```python
from build123d import *

# Parameters (mm, degrees)
BOSS_EXTRUDE1_DEPTH      = 65.5
CUT_EXTRUDE1_DEPTH       = 123.81081001013399
SKETCH5_W                = 286.8159556552996
SKETCH5_H                = 274.5057689508883
CUT_EXTRUDE2_DEPTH       = 124.35386359594037
FILLET1_R                = 1.5
SKETCH6_R                = 1.4499999999976838
SKETCH6_R_2              = 1.4499999999976672
CUT_EXTRUDE3_DEPTH       = 12.7
FILLET2_R                = 1.5
BOSS_EXTRUDE2_DEPTH      = 129.03199999999995
BOSS_EXTRUDE2_DEPTH_BACK = 6.35
FILLET3_R                = 1.5
SKETCH9_R                = 1.4499999999972695
SKETCH9_R_2              = 1.450000000000002
SKETCH9_R_3              = 1.44999999999727
SKETCH9_R_4              = 1.4500000000000004
CUT_EXTRUDE4_DEPTH       = 12.7
CUT_EXTRUDE5_START       = -12.7
SKETCH12_R               = 1.4500000000000008
SKETCH12_R_2             = 1.4499999999999993
SKETCH12_R_3             = 1.450000000000002
CUT_EXTRUDE5_DEPTH       = 12.7


with BuildPart() as part:
    # Sketch2 → Boss-Extrude1 (new body)
    with BuildSketch(Plane.XY):
        Polygon((-105.82469127018673, 132.22169365322222), (-100.10969127018673, 142.12036401847837), (-43.467299735665506, 109.41786401847837), (-49.1822997356655, 99.51919365322226), align=None)
    extrude(amount=BOSS_EXTRUDE1_DEPTH)

    # Sketch4 → Cut-Extrude1 (cut, through all)
    with BuildSketch(Plane(origin=(-102.92764878057318, 59.4253057305198, 68.61843252038122), x_dir=(-0.43301270189221336, 0.2499999999999988, -0.866025403784442), z_dir=(0.750000000000001, -0.4330127018922244, -0.4999999999999942))):
        with BuildLine():
            Line((12.055567275641103, -70.09999999999997), (68.18956727564095, -70.09999999999998))
            ThreePointArc((68.18956727564095, -70.09999999999998), (70.61140800120485, -69.0968407255639), (71.61456727564105, -66.675))
            Line((71.61456727564105, -66.675), (71.61456727564108, 66.67500000000005))
            ThreePointArc((71.61456727564108, 66.67500000000005), (70.611408001205, 69.096840725564), (68.18956727564107, 70.10000000000008))
            Line((68.18956727564107, 70.10000000000008), (12.055567275641172, 70.10000000000008))
            ThreePointArc((12.055567275641172, 70.10000000000008), (9.63372655007727, 69.096840725564), (8.630567275641152, 66.67500000000008))
            Line((8.630567275641152, 66.67500000000008), (8.630567275641091, -66.67499999999998))
            ThreePointArc((8.630567275641091, -66.67499999999998), (9.633726550077167, -69.09684072556392), (12.055567275641103, -70.09999999999997))
        make_face()
    extrude(amount=-CUT_EXTRUDE1_DEPTH, mode=Mode.SUBTRACT)

    # Sketch5 → Cut-Extrude2 (cut, through all)
    with BuildSketch(Plane(origin=(-104.07064878057318, 60.08521708820357, 69.38043252038125), x_dir=(0.43301270189221336, -0.2499999999999988, 0.866025403784442), z_dir=(-0.750000000000001, 0.43301270189222446, 0.4999999999999942))):
        with Locations((-47.42628955617079, -22.345577128817233)):
            Rectangle(SKETCH5_W, SKETCH5_H)
    extrude(amount=CUT_EXTRUDE2_DEPTH, mode=Mode.SUBTRACT)

    # Fillet1
    fillet1_edges = [part.edges().sort_by_distance(p)[0] for p in [
        (-43.467299735665506, 109.41786401847837, 32.75),
        (-84.80402815547504, 133.28363529907386, 34.88867377057616),
        (-76.11182953811208, 115.06696493381483, 63.70307100530266),
        (-49.1822997356655, 99.51919365322226, 32.75),
    ]]
    fillet(fillet1_edges, radius=FILLET1_R)

    # Sketch6 → Cut-Extrude3 (cut)
    with BuildSketch(Plane(origin=(-102.92764878057321, 59.42530573051982, 68.61843252038126), x_dir=(0.4330127018922132, -0.24999999999999897, 0.866025403784442), z_dir=(-0.750000000000001, 0.4330127018922244, 0.4999999999999942))):
        with Locations(Location((-12.4365672756387, 66.29527000000009, 0), (0, 0, 16.102113752))):
            Circle(SKETCH6_R)
        with Locations(Location((-67.80856727563872, 66.29527000000007, 0), (0, 0, 16.102113752))):
            Circle(SKETCH6_R_2)
    extrude(amount=-CUT_EXTRUDE3_DEPTH, mode=Mode.SUBTRACT)

    # Fillet2
    # the kernel refuses this fillet: 1.5 mm, written as the material it takes off along each edge
    with BuildSketch(Plane(origin=(-100.10969127018673, 142.12036401847837, -3.75), x_dir=(-0.5, -0.8660254037844387, 0), z_dir=(0, 0, 1))) as fillet2_piece_1:
        with BuildLine():
            CenterArc((FILLET2_R, FILLET2_R), FILLET2_R, 180, 90)
            Line((3e-17, FILLET2_R), (0, 0))
            Line((0, 0), (FILLET2_R, 0))
        make_face()
    extrude(amount=8.777347541152302, mode=Mode.SUBTRACT)


with BuildPart() as body_2:
    # Mirror2: mirrored copy
    add(part.part.mirror(Plane(origin=(0, 0, 0), x_dir=(1e-16, 1.8e-16, 1), z_dir=(0.500000000000004, 0.8660254037844364, 0))))


with BuildPart() as part_1:
    add(part.part)

    add(body_2.part)  # Boss-Extrude2 merges body 2
    # Sketch8 → Boss-Extrude2 (add, two sides: drawn at the far end of the back side and taken through both)
    with BuildSketch(Plane(origin=(30.797500000000397, 53.34283474610328, 0), x_dir=(0.866025403784437, -0.5000000000000029, 0), z_dir=(-0.5000000000000029, -0.866025403784437, 0)).offset(-BOSS_EXTRUDE2_DEPTH_BACK)):
        Polygon((-154.5827178142381, 6.554994353133541), (-155.97771781422597, 7.360397978646052), (-157.7577178142381, 4.277347541152373), (-157.7577178142381, 0), (-154.58271781423835, 0), align=None)
        Polygon((-123.18667970854972, 61.15614201060529), (-121.73608733433291, 60.31864170382078), (-118.74462872726596, 65.50000000000001), (-120.67875212905116, 65.50000000000001), (-122.41080293662007, 65.50000000000001), (-124.48571781422638, 61.90614201060528), align=None)
    extrude(amount=BOSS_EXTRUDE2_DEPTH + BOSS_EXTRUDE2_DEPTH_BACK)

    # Fillet3
    fillet3_edges = [part_1.edges().sort_by_distance(p)[0] for p in [
        (-172.53112429253738, 15.785626111925975, 4.1571540602531725),
        (-136.62219127018705, 78.87885890711985, 4.277347541152341),
        (-99.93631537383828, 141.5235235248658, 4.157154060253142),
    ]]
    fillet(fillet3_edges, radius=FILLET3_R)

    # Sketch9 → Cut-Extrude4 (cut)
    with BuildSketch(Plane.XY.offset(65.50000000000001)):
        with Locations((-67.1597126180574, 116.49757139704164)):
            Circle(SKETCH9_R)
        with Locations((-49.7889013508033, 106.4685288358503)):
            Circle(SKETCH9_R_2)
        with Locations((-134.46971261805777, -0.08676846042013409)):
            Circle(SKETCH9_R_3)
        with Locations((-117.0989013508037, -10.115811021611455)):
            Circle(SKETCH9_R_4)
    extrude(amount=-CUT_EXTRUDE4_DEPTH, mode=Mode.SUBTRACT)

    # Sketch12 → Cut-Extrude5 (cut)
    with BuildSketch(Plane(origin=(0, 0, 0), x_dir=(-1, 0, 0), z_dir=(0, 0, -1)).offset(CUT_EXTRUDE5_START)):
        with Locations((163.84262252006926, 16.871688978388832)):
            Circle(SKETCH12_R)
        with Locations(Location((117.09890135080418, -10.115811021611187, 0), (0, 0, 180))):
            Circle(SKETCH12_R_2)
        with Locations((96.53262252006812, 133.4560288358508)):
            Circle(SKETCH12_R_3)
        with Locations(Location((49.78890135080324, 106.46852883585038, 0), (0, 0, 180))):
            Circle(SKETCH12_R_3)
    extrude(amount=CUT_EXTRUDE5_DEPTH, mode=Mode.SUBTRACT)


solid = part_1.part
```
Design review of the part built by this model. Coordinates are the model's own, in mm. A direction names the side the tool comes from. Give positions to 0.01 mm unless a question says otherwise; leave off trailing zeros. Return JSON: item names as keys, results as strings. Group by question number.
(1) Insertion check: pin 1 (5 mm diameter, centred on x = -121.5, z = 35, fed in from +Y); pin 2 (4.5 mm diameter, centred on x = -96.53, y = 133.46, fed in from -Z); pin 3 (2.5 mm diameter, centred on x = -117.1, y = -10.12, fed in from -Z); pin 4 (12 mm diameter, centred on x = -82, z = 8, fed in from +Y). Each pin has a flat end and moves straight along its axis. Give the tip position at first contact, or say it passes through.
(2) We need section A-A, the plane x = -92.5. Give the number of separate pieces and of enclosed holes in the cut face, then the cut area to 3 significant figures.
(3) To check wall thickness, follow probe 1 along Y at (x, z) = (-113, 6.5); probe 2 along X at (y, z) = (8, 25.5); probe 3 along Y at (x, z) = (-123.5, 32). State the ranges of each line that lie inside material, in increasing order.
(4) Mouldability with a two-part tool opening along Z and no side actions: class faces 1 (the cylindrical face through (-95.131, 129.804, 6.842)), 2 (the flat face through (-103.72, 60.88, 62.87)), 3 (the flat face through (-137.123, 78.012, 1.911)) as +Z half, -Z half, draft (parallel to the pull), parting line (faces both ways), or undercut.
(5) Machinability: for faces 4 (the flat face through (-70.59, 111.88, 25.01)), 5 (the cylindrical face through (-73.113, 122.028, 60.628)), 6 (the cylindrical face through (-168.6, 17.6, 7.8)), which of the approach directions +Z, -Z, +X, -X, +Y, -Y give a long, thin tool a straight path to every point of the face, cutting with its end or side? Answer none if there is none.
Reported:
{
 "1": {"pin 1": "stops at y = 0.47", "pin 2": "stops at z = 0", "pin 3": "stops at z = 12.7", "pin 4": "stops at y = 135.13"},
 "2": {"separate pieces": "2", "enclosed holes": "1", "area": "325 mm2"},
 "3": {"probe 1": "y = -11.02 to -5.88, 113.44 to 117.23", "probe 2": "x = -159.91 to -137.05", "probe 3": "y = -13.02 to 0.18"},
 "4": {"face 1": "undercut", "face 2": "-Z half", "face 3": "draft"},
 "5": {"face 4": "-Z, -Y", "face 5": "-X", "face 6": "+Z"}
}
